Model file for the job. Use its own axes, mm. Give positions to 0.01 mm unless a question says otherwise; leave off trailing zeros. Order: outer loops, then holes, each group sorted by start corner. A loop starts at its lowest first (then second) coordinate and runs counter-clockwise, first axis right, second up. Notation, with made-up numbers: M 39.5,35.5 L 93.5,35.5 A21 ccw 93.5,70.5 Z; hole C -2,1.5 d1. An arc over 180 degrees is marked long. Return JSON: item names as keys, results as strings. Group by question number.
1. Slice it at D-D on z = -40. List the corners of the cut face in (x, y), then the cut area to 3 significant figures.
2. Slice it at B-B on x = 10.85. List the corners of the cut face in (y, z).
3. Pin check, flat tips, straight feed: pin 1 (2.5 mm diameter, centred on x = 61.65, z = -47, fed in from -Y); pin 2 (4.5 mm diameter, centred on x = 10.85, z = -47, fed in from +Y); pin 3 (0.8 mm diameter, centred on y = 10.5, z = -29, fed in from +X). Stop position of each tip, or through.
4. Wall check: probe 1 along X at (y, z) = (2.25, -12.5); probe 2 along Z at (x, y) = (61.65, 3.75); probe 3 along Z at (x, y) = (63, 0.75). Give the ranges that are in metal, low to high. Write a range as [from, to].
5. Slice it at C-C on x = 35. List the corners of the cut face in (y, z).
6. Slice it at A-A on z = -12.5. List the corners of the cut face in (x, y).
from build123d import *

# Parameters (mm, degrees)
SKETCH1_W                  = 72.5
SKETCH1_H                  = 59.5
BOSS_EXTRUDE1_DEPTH        = 10
SKETCH4_W                  = 66
SKETCH4_H                  = 11.5
BOSS_EXTRUDE3_DEPTH        = 1
TAP_DRILL_FOR_10_24_TAP1_D = 3.7973


with BuildPart() as part:
    # Sketch1 → Boss-Extrude1 (new body)
    with BuildSketch(Plane(origin=(0, 0, 0), x_dir=(1, 0, 0), z_dir=(0, 1, 0))):
        with Locations((36.25, 29.75)):
            Rectangle(SKETCH1_W, SKETCH1_H)
    extrude(amount=BOSS_EXTRUDE1_DEPTH)

    # Sketch4 → Boss-Extrude3 (add)
    with BuildSketch(Plane(origin=(0, 10, 0), x_dir=(1, 0, 0), z_dir=(0, 1, 0))):
        with Locations((36.25, 29.75)):
            Rectangle(SKETCH4_W, SKETCH4_H)
    extrude(amount=BOSS_EXTRUDE3_DEPTH)

    # Tap Drill for #10-24 Tap1 (through all)
    with Locations(Plane(origin=(0, 10, 0), x_dir=(1, 0, 0), z_dir=(0, 1, 0))):
        with Locations((10.85, 47), (61.65, 47), (10.85, 12.5), (61.65, 12.5)):
            Hole(TAP_DRILL_FOR_10_24_TAP1_D / 2)


solid = part.part
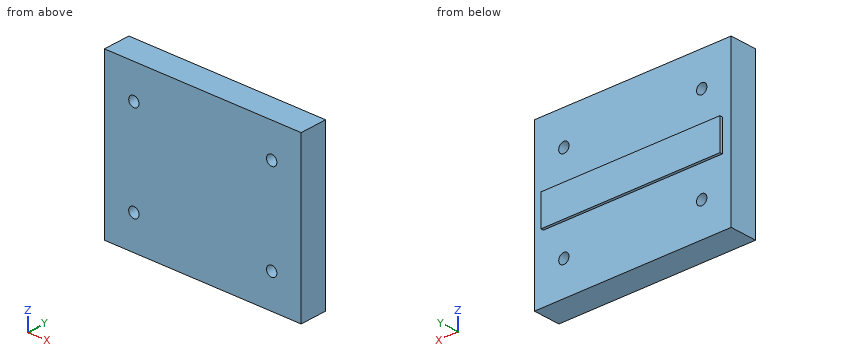
Result:
{
 "1": {"outline": "M 0,0 L 72.5,0 L 72.5,10 L 0,10 Z", "area": "725 mm2"},
 "2": {"outline": "M 0,-59.5 L 10,-59.5 L 10,-48.9 L 0,-48.9 Z; M 0,-45.1 L 10,-45.1 L 10,-35.5 L 11,-35.5 L 11,-24 L 10,-24 L 10,-14.4 L 0,-14.4 Z; M 0,-10.6 L 10,-10.6 L 10,0 L 0,0 Z"},
 "3": {"pin 1": "passes through", "pin 2": "stops at y = 10", "pin 3": "stops at x = 69.25"},
 "4": {"probe 1": "x = [0, 8.95], [12.75, 59.75], [63.55, 72.5]", "probe 2": "z = [-59.5, -48.9], [-45.1, -14.4], [-10.6, 0]", "probe 3": "z = [-59.5, -48.34], [-45.66, -13.84], [-11.16, 0]"},
 "5": {"outline": "M 0,-59.5 L 10,-59.5 L 10,-35.5 L 11,-35.5 L 11,-24 L 10,-24 L 10,0 L 0,0 Z"},
 "6": {"outline": "M 0,0 L 8.95,0 L 8.95,10 L 0,10 Z; M 12.75,0 L 59.75,0 L 59.75,10 L 12.75,10 Z; M 63.55,0 L 72.5,0 L 72.5,10 L 63.55,10 Z"}
}
